Autodesk Inventor part; units mm, degrees
ref_plane "YZ Plane" through (0, 0, 0) normal (1, 0, 0) x (0, 1, 0)
ref_plane "XZ Plane" through (0, 0, 0) normal (0, 1, 0) x (-1, 0, 0)
ref_plane "XY Plane" through (0, 0, 0) normal (0, 0, 1) x (1, 0, 0)
sketch "Sketch1" plane through (0, 0, 0) normal (0, 0, 1) x (1, 0, 0)
  line L0 (0, 0) -> (0, 150)
  line L1 (46.5, 103.1016) -> (49.5, 103.1016)
  line L2 (49.5, 103.1016) -> (49.5, 4.6016)
  line L3 (48, 3.1016) -> (48, 3.1016)
  line L4 (46.5, 4.6016) -> (46.5, 103.1016)
  line L5 (49.5, 48.1016) -> (51.75, 48.1016)
  line L6 (51.75, 48.1016) -> (51.75, 53.1016)
  line L7 (51.75, 53.1016) -> (49.5, 53.1016)
  line L8 (49.5, 53.1016) -> (49.5, 48.1016)
  arc A0 (46.5, 4.6016) -> (48, 3.1016) centre (48, 4.6016) ccw
  arc A1 (48, 3.1016) -> (49.5, 4.6016) centre (48, 4.6016) ccw
  point P0 (49.5, 3.1016)
  point P1 (46.5, 3.1016)
  dimension "d1" = 100
  dimension "d2" = 50
  dimension "d3" = 5
  dimension "d4" = 3
  dimension "d5" = 99
  dimension "d6" = 103.5
  dimension "d8" = 1.5
revolve "Revolution1" add sketch "Sketch1" angle 360 about axis through (0, 0, 0) along (0, 1, 0)
properties part number "pld_bh"
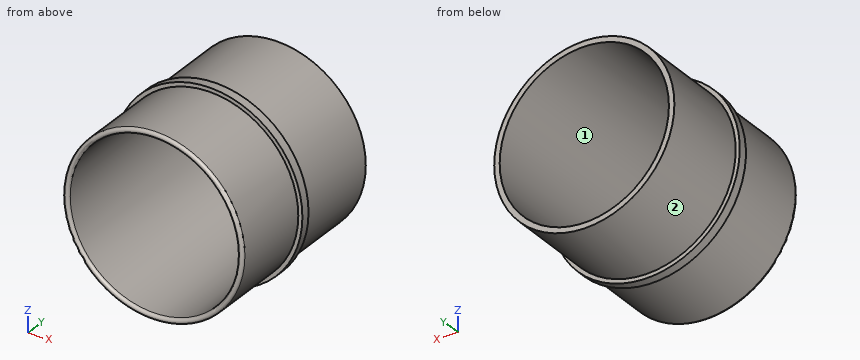
Verification items for the finished model (mm, model axes). Face numbers are marked on the shaded views. Round coordinates to 2 decimals unless told otherwise and drop trailing zeros. Order: outer loops, then holes, each group sorted by start corner. A loop starts at its lowest first (then second) coordinate and runs counter-clockwise, first axis right, second up.
1. Release check for a two-part mould opening along X. For the marked faces 1 and 2 record: +X half, -X half, draft (parallel to the pull), parting line (faces both ways), or undercut.
Final values:
face 1: undercut
face 2: parting line
2. Section check B-B on x = 0. Record the cut outline in (y, z).
Final values:
outline: (4.6, -49.5) - (48.1, -49.5) - (48.1, -51.75) - (53.1, -51.75) - (53.1, -49.5) - (103.1, -49.5) - (103.1, -46.5) - (4.6, -46.5) arc R1.5 ccw to start; (4.6, 46.5) - (103.1, 46.5) - (103.1, 49.5) - (53.1, 49.5) - (53.1, 51.75) - (48.1, 51.75) - (48.1, 49.5) - (4.6, 49.5) arc R1.5 ccw to start
3. Go/stop test with flat-tipped pins: P1, Ø6, axis at x = -30.5, y = 75.5, coming from the +Z side; P2, Ø2, axis at x = -1, y = 14.5, coming from the -Z side; P3, Ø4, axis at x = -40, z = 22, coming from the +Y side; P4, Ø8, axis at y = 93, z = -20, coming from the +X side. Record where each tip stops, or that it passes through.
Final values:
P1: stops at z = 41.16
P2: stops at z = -49.5
P3: stops at y = 103.1
P4: stops at x = 46.84
4. Section check A-A on z = 0. Record the cut outline in (x, y), then the cut area to 3 significant figures.
Final values:
outline: (-51.75, 48.1) - (-49.5, 48.1) - (-49.5, 4.6) arc R1.5 ccw to (-46.5, 4.6) - (-46.5, 103.1) - (-49.5, 103.1) - (-49.5, 53.1) - (-51.75, 53.1) - close; (46.5, 4.6) arc R1.5 ccw to (49.5, 4.6) - (49.5, 48.1) - (51.75, 48.1) - (51.75, 53.1) - (49.5, 53.1) - (49.5, 103.1) - (46.5, 103.1) - close
area: 621 mm2
5. Thickness scan on L1, parallel to X at y = 74.5, z = 0; L2, parallel to Z at x = 0, y = 49. Record the ranges inside material, lowest first.
Final values:
L1: x = -49.5 to -46.5, 46.5 to 49.5
L2: z = -51.75 to -46.5, 46.5 to 51.75
6. Section check C-C on y = 74. Record the cut outline in (x, z).
Final values:
outline: circle Ø99 at (0, 0); hole circle Ø93 at (0, 0)
